Here's how the part is built. I have some questions about the finished solid (model axes, mm). Face numbers are marked on the shaded views. A direction names the side the tool comes from. Coordinates: 2 decimals unless noted, no trailing zeros. Write each loop counter-clockwise with the first axis right and the second up, starting at its lowest first coordinate (ties: lowest second). Pieces come first, ordered by that corner, then holes. Notation, with made-up numbers: M 75.25,-20 L 99.25,-20 A18 cw 99.25,-13 Z; hole C -19.75,5.5 d11. An arc over 180 degrees is marked long. Use a Markdown table: item, result.
Autodesk Fusion 360 part; units mm, degrees
sketch "Sketch1" plane through (0, 0, 0) normal (0, 0, 1) x (1, 0, 0)
  line L0 (0, 0) -> (26, 0)
  line L1 (26, 0) -> (26, 36)
  line L2 (26, 36) -> (0, 36)
  line L3 (0, 36) -> (0, 0)
  line L4 (3, 3) -> (23, 3)
  line L5 (3, 33) -> (3, 3)
  line L6 (23, 3) -> (23, 33)
  line L7 (23, 33) -> (3, 33)
  dimension "d2" = 30
sketch "Sketch3" plane through (0, 0, 0) normal (0, 0, 1) x (1, 0, 0)
  line L0 (12, 33) -> (14, 33)
  line L1 (14, 33) -> (14, 3)
  line L2 (14, 3) -> (12, 3)
  line L3 (12, 3) -> (12, 33)
  line L4 (23, 19) -> (3, 19)
  line L5 (3, 19) -> (3, 17)
  line L6 (3, 17) -> (23, 17)
  line L7 (23, 17) -> (23, 19)
extrude "Extrude1" add sketch "Sketch1" along normal blind 4
extrude "Extrude5" add sketch "Sketch3" along normal blind 4 contours L0 L1 L3 L4 | L1 L3 L4 L6 | L1 L2 L3 L6
extrude "Extrude6" add sketch "Sketch3" along normal blind 4 contours L3 L4 L5 L6
extrude "Extrude7" add sketch "Sketch3" along normal blind 4 contours L1 L4 L6 L7
sketch "Sketch5" plane through (0, 0, 0) normal (0, 0, 1) x (1, 0, 0)
  line L0 (26, 36) -> (0, 36)
  line L1 (0, 0) -> (26, 0)
  line L2 (0, 36) -> (0, 0)
  line L3 (26, 0) -> (26, 36)
extrude "Extrude9" add sketch "Sketch5" along normal blind 1
sketch "Sketch6" plane through (0, 0, 4) normal (0, 0, 1) x (-1, 0, 0)
  line L0 (-14, -19) -> (-14, -33)
  line L1 (-14, -33) -> (-23, -33)
  line L2 (-23, -33) -> (-23, -19)
  line L3 (-23, -19) -> (-14, -19)
  line L4 (-3, -19) -> (-3, -33)
  line L5 (-3, -33) -> (-12, -33)
  line L6 (-12, -33) -> (-12, -19)
  line L7 (-12, -19) -> (-3, -19)
  line L8 (-14, -17) -> (-23, -17)
  line L9 (-23, -17) -> (-23, -3)
  line L10 (-23, -3) -> (-14, -3)
  line L11 (-14, -3) -> (-14, -17)
  line L12 (-3, -17) -> (-12, -17)
  line L13 (-12, -17) -> (-12, -3)
  line L14 (-12, -3) -> (-3, -3)
  line L15 (-3, -3) -> (-3, -17)
  line L16 (0, -36) -> (0, 0)
  line L17 (0, 0) -> (-26, 0)
  line L18 (-26, 0) -> (-26, -36)
  line L19 (-26, -36) -> (0, -36)
extrude "Extrude10" cut sketch "Sketch6" against normal blind 0.75
extrude "Extrude8" [suppressed]
extrude "Extrude4" [suppressed]
extrude "Extrude3" [suppressed]
extrude "Extrude2" [suppressed]
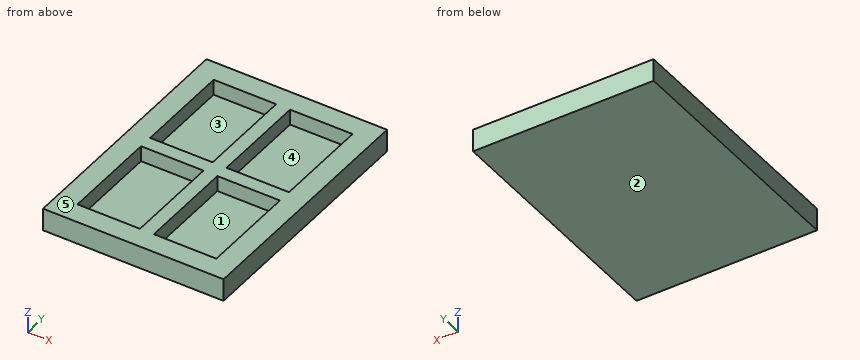
1. Suppose I cut it at A-A on y = 26. Write out the boundary of the cut face in (x, z).
Answers follow:
| item | result |
|---|---|
| outline | M 0,0 L 26,0 L 26,3.25 L 23,3.25 L 23,1 L 14,1 L 14,3.25 L 12,3.25 L 12,1 L 3,1 L 3,3.25 L 0,3.25 Z |
2. Suppose I cut it at B-B on x = 6. Write out the boundary of the cut face in (y, z).
Answers follow:
| item | result |
|---|---|
| outline | M 0,0 L 36,0 L 36,3.25 L 33,3.25 L 33,1 L 19,1 L 19,3.25 L 17,3.25 L 17,1 L 3,1 L 3,3.25 L 0,3.25 Z |
3. I need wall thicknesses on probe 1 along X at (y, z) = (16.5, 2.4); probe 2 along Y at (x, z) = (20.5, 2.6); probe 3 along Z at (x, y) = (17.75, 10.5). Which ranges of each line are inside material? Lowest first, please.
Answers follow:
| item | result |
|---|---|
| probe 1 | x = 0 to 3, 12 to 14, 23 to 26 |
| probe 2 | y = 0 to 3, 17 to 19, 33 to 36 |
| probe 3 | z = 0 to 1 |
4. Suppose I cut it at C-C on z = 2.55. Write out the boundary of the cut face in (x, y), and give its area (3 significant figures).
Answers follow:
| item | result |
|---|---|
| outline | M 0,0 L 26,0 L 26,36 L 0,36 Z; hole M 3,3 L 12,3 L 12,17 L 3,17 Z; hole M 3,19 L 12,19 L 12,33 L 3,33 Z; hole M 14,3 L 23,3 L 23,17 L 14,17 Z; hole M 14,19 L 23,19 L 23,33 L 14,33 Z |
| area | 432 mm2 |
5. Which directions (+Z, -Z, +X, -X, +Y, -Y) give clear straight access to the entire face, cutting with the end or side of a thin tool? Please do the marked faces 1 and 2.
Answers follow:
| item | result |
|---|---|
| face 1 | +Z |
| face 2 | -Z, +X, -X, +Y, -Y |
6. We'd pull the mould along X, two halves only. Please class the marked faces 3, 4 and 5: +X half, -X half, draft (parallel to the pull), parting line (faces both ways), or undercut.
Answers follow:
| item | result |
|---|---|
| face 3 | undercut |
| face 4 | undercut |
| face 5 | draft |
